Can you work these out from the model? Positions are in its coordinate system, mm. A direction names the side the tool comes from. Give positions to 0.01 mm unless a question says otherwise; leave off trailing zeros. Order: outer loops, then holes, each group sorted by start corner. A loop starts at its lowest first (then second) coordinate and runs counter-clockwise, first axis right, second up. Notation, with made-up numbers: M -37,82.25 L 0,82.25 A15 cw 0,95.25 Z; hole C -5.5,70 d3. An arc over 180 degrees is marked long. Write each question's results on one line, items separated by ' | '.
from build123d import *

# Parameters (mm, degrees)
EXTRUDE_1_DEPTH     = 4
SKETCH_2_R          = 1.5
CUT_EXTRUDE_1_DEPTH = 4
SKETCH_3_W          = 10
SKETCH_3_H          = 69.678883607
SKETCH_3_H_2        = 93.047687854
CUT_EXTRUDE_2_DEPTH = 4
CUT_EXTRUDE_3_DEPTH = 4


with BuildPart() as part:
    # 草图1 → 凸台-拉伸1 (new body)
    with BuildSketch(Plane(origin=(0, 0, 0), x_dir=(1, 0, 0), z_dir=(0, 1, 0))):
        Polygon((-67.5, -35), (-47.5, -15), (2.5, -15), (22.5, -35), (92.5, -35), (92.5, 15), (72.5, 35), (-117.5, 35), (-137.5, 15), (-137.5, -35), align=None)
    extrude(amount=EXTRUDE_1_DEPTH)

    # 草图2 → 切除-拉伸1 (cut)
    with BuildSketch(Plane(origin=(0, 4, 0), x_dir=(1, 0, 0), z_dir=(0, 1, 0))):
        with Locations(Location((-97.5, -15, 0), (0, 0, 270))):
            Circle(SKETCH_2_R)
        with Locations(Location((-97.5, 25, 0), (0, 0, 270))):
            Circle(SKETCH_2_R)
        with Locations(Location((52.5, 25, 0), (0, 0, 90))):
            Circle(SKETCH_2_R)
        with Locations(Location((52.5, -15, 0), (0, 0, 90))):
            Circle(SKETCH_2_R)
    extrude(amount=-CUT_EXTRUDE_1_DEPTH, mode=Mode.SUBTRACT)

    # 草图3 → 切除-拉伸2 (cut)
    with BuildSketch(Plane(origin=(0, 4, 0), x_dir=(1, 0, 0), z_dir=(0, 1, 0))):
        with Locations((-132.5, -0.160558196)):
            Rectangle(SKETCH_3_W, SKETCH_3_H)
        with Locations((87.5, 11.523843927)):
            Rectangle(SKETCH_3_W, SKETCH_3_H_2)
    extrude(amount=-CUT_EXTRUDE_2_DEPTH, mode=Mode.SUBTRACT)

    # 草图4 → 切除-拉伸3 (cut)
    with BuildSketch(Plane(origin=(0, 4, 0), x_dir=(1, 0, 0), z_dir=(0, 1, 0))):
        Polygon((-127.5, 12.5), (-92.197077218, 47.802922782), (-150.178982695, 47.802922782), align=None)
        Polygon((82.5, 12.5), (37.005283765, 57.994716235), (96.544114713, 56.205234398), align=None)
    extrude(amount=-CUT_EXTRUDE_3_DEPTH, mode=Mode.SUBTRACT)


solid = part.part
(1) I need wall thicknesses on L1, parallel to Z at x = 52.5, y = 2.85; L2, parallel to X at y = 1, z = -25; L3, parallel to X at y = 1.55, z = 32. Which ranges of each line are inside material? Lowest first, please. Write a range as from..to.
Data:
L1: z = -35..-26.5, -23.5..13.5, 16.5..35 | L2: x = -115..-99, -96..51, 54..70 | L3: x = -127.5..-64.5, 19.5..82.5
(2) Imagine slicing it at C-C, the plane z = -20.5. Write out the boundary of the cut face in (x, y), plus the area to 3 significant figures.
Data:
outline: M -119.5,0 L 74.5,0 L 74.5,4 L -119.5,4 Z | area: 776 mm2
(3) Imagine slicing it at A-A, the plane y = 2.9. Write out the boundary of the cut face in (x, z).
Data:
outline: M -127.5,-12.5 L -105,-35 L 60,-35 L 82.5,-12.5 L 82.5,35 L 22.5,35 L 2.5,15 L -47.5,15 L -67.5,35 L -127.5,35 Z; hole C -97.5,-25 d3; hole C -97.5,15 d3; hole C 52.5,-25 d3; hole C 52.5,15 d3
(4) For faces 1 (the face through (-57.6, 2, 25.1)), 2 (the face through (82.5, 2, 12)), which set-ups out of +Z, -Z, +X, -X, +Y, -Y let a thin tool reach every point of the face, with its end or its side?
Data:
face 1: +Z, +Y, -Y | face 2: +Z, -Z, +X, +Y, -Y
(5) Imagine slicing it at B-B, the plane x = -37.5. Write out the boundary of the cut face in (y, z), plus the area to 3 significant figures.
Data:
outline: M 0,-35 L 4,-35 L 4,15 L 0,15 Z | area: 200 mm2
(6) Will these pins go through, and if not, where does the flat tip stop? P1, Ø5, axis at x = 53, z = 17.5, coming from the -Y side; P2, Ø2.5, axis at x = 52.5, z = -25, coming from the +Y side; P3, Ø2, axis at x = -28, y = 2.5, coming from the +Z side.
Data:
P1: stops at y = 0 | P2: passes through | P3: stops at z = 15
